```python
from build123d import *

# Parameters (mm, degrees)
SKETCH1_W           = 1676.4
SKETCH1_H           = 165.1
BOSS_EXTRUDE1_DEPTH = 165.1
SKETCH2_W           = 139.7
SKETCH2_H           = 139.7
CUT_EXTRUDE1_DEPTH  = 1676.4
SKETCH4_R           = 6.35
CUT_EXTRUDE3_DEPTH  = 12.7


with BuildPart() as part:
    # Sketch1 → Boss-Extrude1 (new body)
    with BuildSketch(Plane.XY):
        with Locations((838.2, 82.55)):
            Rectangle(SKETCH1_W, SKETCH1_H)
    extrude(amount=BOSS_EXTRUDE1_DEPTH)

    # Sketch2 → Cut-Extrude1 (cut)
    with BuildSketch(Plane(origin=(1676.4, 0, 0), x_dir=(0, 0, -1), z_dir=(1, 0, 0))):
        with Locations((-82.55, 82.55)):
            Rectangle(SKETCH2_W, SKETCH2_H)
    extrude(amount=-CUT_EXTRUDE1_DEPTH, mode=Mode.SUBTRACT)

    # Sketch4 → Cut-Extrude3 (cut)
    with BuildSketch(Plane(origin=(0, 165.1, 0), x_dir=(1, 0, 0), z_dir=(0, 1, 0))):
        with Locations((38.1, -82.55)):
            Circle(SKETCH4_R)
        with Locations((1638.3, -82.55)):
            Circle(SKETCH4_R)
    extrude(amount=-CUT_EXTRUDE3_DEPTH, mode=Mode.SUBTRACT)


solid = part.part
```
Here's how the part is built. I have some questions about the finished solid (model axes, mm). A direction names the side the tool comes from. Coordinates: 2 decimals unless noted, no trailing zeros. Order: outer loops, then holes, each group sorted by start corner. A loop starts at its lowest first (then second) coordinate and runs counter-clockwise, first axis right, second up.
Item 1: If we section it at A-A, the plane y = 49.5: List the corners of the cut face in (x, z) for me, then the cut area to 3 significant figures.
Response values:
outline: (0, 0) - (1676.4, 0) - (1676.4, 12.7) - (0, 12.7) - close; (0, 152.4) - (1676.4, 152.4) - (1676.4, 165.1) - (0, 165.1) - close
area: 42,600 mm2
Item 2: I'm going to push a flat-ended pin straight in: pin 1 Ø10 at (x, z) = (1638.3, 82.55) entering from +Y. Where does the tip first touch, or does it pass through?
Response values:
pin 1: stops at y = 12.7
Item 3: If we section it at B-B, the plane x = 184.5: List the corners of the cut face in (y, z) for me, then the cut area to 3 significant figures.
Response values:
outline: (0, 0) - (165.1, 0) - (165.1, 165.1) - (0, 165.1) - close; hole (12.7, 12.7) - (152.4, 12.7) - (152.4, 152.4) - (12.7, 152.4) - close
area: 7,740 mm2
Item 4: Which directions (+Z, -Z, +X, -X, +Y, -Y) give clear straight access to the entire face, cutting with the end or side of a thin tool? Please do faces 1 (the face through (1676.4, 8, 81)), 2 (the face through (850, 82, 12.7)).
Response values:
face 1: +Z, -Z, +X, +Y, -Y
face 2: +X, -X
Item 5: I need wall thicknesses on probe 1 along X at (y, z) = (160.25, 82.55); probe 2 along Z at (x, y) = (733.5, 133). Which ranges of each line are inside material? Lowest first, please.
Response values:
probe 1: x = 0 to 31.75, 44.45 to 1631.95, 1644.65 to 1676.4
probe 2: z = 0 to 12.7, 152.4 to 165.1
Item 6: Thinking about a two-plate mould opening in Y: for faces 3 (the face through (0, 8, 81)), 4 (the face through (826, 0, 81)), 5 (the face through (850, 82, 152.4)), which applies, pulls with the +Y half, pulls with the -Y half, needs draft (parallel to the pull), parting line crosses it, or undercut?
Response values:
face 3: needs draft
face 4: pulls with the -Y half
face 5: undercut
